Design review of the part built by this model. Coordinates are the model's own, in mm. Give positions to 0.01 mm unless a question says otherwise; leave off trailing zeros. Loops run counter-clockwise (first coordinate to the right, second up) from the corner with the lowest first, then second, coordinate; pieces in that order, holes last. Notation, with made-up numbers: (-24, -3) -> (25, -3) arc R32 cw to (25, 29) -> close; hole circle Ø4 at (-23.75, -29.75). An arc over 180 degrees is marked (long way). Answer as CSV lines item,"result".
Autodesk Inventor part; units mm, degrees
ref_plane "工作平面1" through (10, 19, 0) normal (-0.4103, -0.6448, -0.6448) x (0.8437, 0, -0.5369)
ref_plane "YZ Plane" through (0, 0, 0) normal (1, 0, 0) x (0, 1, 0)
ref_plane "XZ Plane" through (0, 0, 0) normal (0, 1, 0) x (-1, 0, 0)
sketch "草圖1" plane through (0, 0, 0) normal (0, 1, 0) x (-1, 0, 0)
  line L0 (0, 0) -> (-54, 0)
  line L1 (-54, 0) -> (-54, -38)
  line L2 (-54, -38) -> (0, -38)
  line L3 (0, -38) -> (0, 0)
  dimension "d0" = 54
  dimension "d1" = 38
extrude "擠出1" add sketch "草圖1" along normal mid plane 38
sketch "草圖2" plane through (0, 19, 0) normal (0, 1, 0) x (1, 0, 0)
  line L0 (0, 0) -> (54, 0)
  line L1 (10, 0) -> (54, 8)
  line L2 (54, 0) -> (54, 38)
  dimension "d4" = 10
  dimension "d5" = 30
extrude "擠出2" cut sketch "草圖2" against normal blind 40
sketch "草圖3" plane through (54, -19, -38) normal (1, 0, 0) x (0, 0, -1)
  line L0 (-30, 18) -> (-10, 38)
  line L1 (0, 38) -> (-38, 38)
  line L2 (-30, 38) -> (-30, 0)
  point P0 (-38, 19)
  dimension "d8" = 20
  dimension "d9" = 20
ref_plane "工作平面1" through (10, 19, 0) normal (-0.4103, -0.6448, -0.6448) x (0.8437, 0, -0.5369)
sketch "草圖4" plane through (10, 19, 0) normal (-0.4103, -0.6448, -0.6448) x (0.8437, 0, -0.5369)
  line L0 (-15.1543, -12.3218) -> (93.717, -12.3218)
  line L1 (93.717, -12.3218) -> (93.717, 28.8166)
  line L2 (93.717, 28.8166) -> (-15.1543, 28.8166)
  line L3 (-15.1543, 28.8166) -> (-15.1543, -12.3218)
  point P0 (-8.4366, 11.0602)
extrude "擠出3" cut sketch "草圖4" against normal blind 40
mirror "鏡射1" about plane through (0, 0, 0) normal (0, 1, 0) of "擠出3"
properties part number "26"
Q1. We need section A-A, the plane z = -19. State the section outline as (x, y) points.
Filled sheet:
outline,"(0, -19) -> (39.85, -19) -> (54, -10) -> (54, 10) -> (39.85, 19) -> (0, 19) -> close"
Q2. Clearance check with a flat-ended pin moving along its axis: pin 1 Ø1 at (x, y) = (46, 2.5) entering from +Z. State where the tip first meets the part, or that it passes through.
Filled sheet:
pin 1,"stops at z = -6.45"
Q3. To check wall thickness, follow probe 1 along Z at (x, y) = (14, -14); probe 2 along Z at (x, y) = (44.5, 4.5); probe 3 along X at (y, z) = (17, -26). State the ranges of each line that lie inside material, in increasing order. Write a range as from..to.
Filled sheet:
probe 1,"z = -38..-0.73"
probe 2,"z = -38..-7.46"
probe 3,"x = 0..54"
Q4. We need section B-B, the plane x = 20.5. State the section outline as (y, z) points.
Filled sheet:
outline,"(-19, -38) -> (19, -38) -> (19, -6.68) -> (14.22, -1.91) -> (-14.22, -1.91) -> (-19, -6.68) -> close"
